Study the drawing (mm; zero at the part's minimum x, y, z) and answer. Round coordinates to 2 decimals unless told otherwise and drop trailing zeros. Write each loop counter-clockwise with the first axis right and the second up, starting at its lowest first coordinate (ties: lowest second). Pieces come first, ordered by that corner, then holes. Notation, with made-up numbers: (-2.75, -4.5) - (4.25, -4.5) arc R15 ccw to (4.25, 8.5) - close; hole circle Ø3 at (73.25, -4). An arc over 180 degrees is marked (long way). Return JSON: item names as keys, results as strings. Group by question number.
(1) Find the intervals of material crossed by line 1 along Z through (x, y) = (49.4, 3.05); line 2 along Z through (x, y) = (49.4, 1.95); line 3 along X through (y, z) = (1.95, 51), in increasing order. Write a range as [from, to].
(2) Section A-A, the plane x = 4 is taken. Write down the section's boundary in (y, z).
(3) Section D-D, the plane x = 16.5 is taken. Write down the section's boundary in (y, z), then the cut area to 3 significant figures.
(4) Section C-C, the plane x = 49.4 is taken. Write down the section's boundary in (y, z), then the cut area to 3 significant figures.
(5) Each of these flat-tipped pins is pushed along its axis until it touches: pin 1 (3.5 mm diameter, centred on x = 49.4, z = 55.8, fed in from +Y); pin 2 (8 mm diameter, centred on x = 47, z = 43.5, fed in from -Y); pin 3 (0.6 mm diameter, centred on x = 2, y = 3, fed in from +Z); pin 4 (0.8 mm diameter, centred on y = 2.5, z = 55, fed in from -X). Where does it stop, or does it pass through?
(6) Section B-B, the plane z = 27.5 is taken. Write down the section's boundary in (x, y), then the cut area to 3 significant figures.
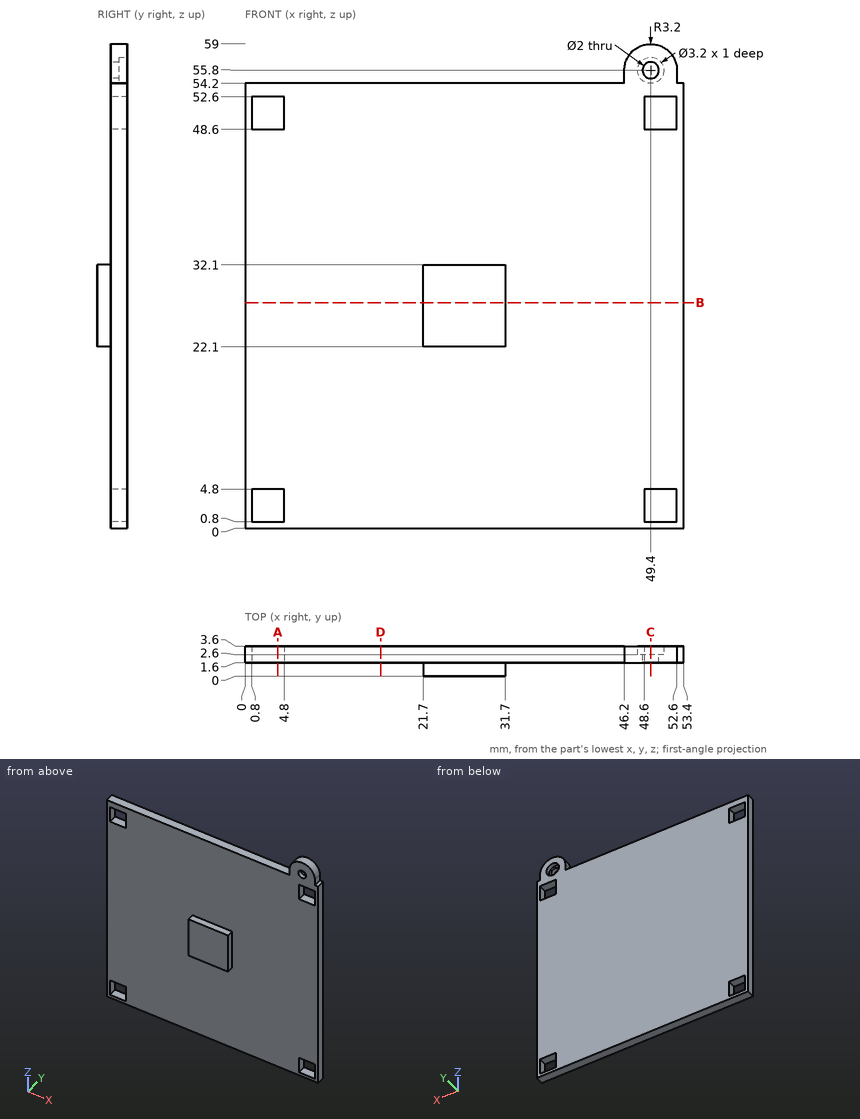
Working result:
{
 "1": {"line 1": "z = [0, 0.8], [4.8, 48.6], [52.6, 54.2], [57.4, 59]", "line 2": "z = [0, 0.8], [4.8, 48.6], [52.6, 54.8], [56.8, 59]", "line 3": "x = [0, 0.8], [4.8, 48.6], [52.6, 53.4]"},
 "2": {"outline": "(1.6, 0) - (3.6, 0) - (3.6, 0.8) - (1.6, 0.8) - close; (1.6, 4.8) - (3.6, 4.8) - (3.6, 48.6) - (1.6, 48.6) - close; (1.6, 52.6) - (3.6, 52.6) - (3.6, 54.2) - (1.6, 54.2) - close"},
 "3": {"outline": "(1.6, 0) - (3.6, 0) - (3.6, 54.2) - (1.6, 54.2) - close", "area": "108 mm^2"},
 "4": {"outline": "(1.6, 0) - (3.6, 0) - (3.6, 0.8) - (1.6, 0.8) - close; (1.6, 4.8) - (3.6, 4.8) - (3.6, 48.6) - (1.6, 48.6) - close; (1.6, 52.6) - (3.6, 52.6) - (3.6, 54.2) - (2.6, 54.2) - (2.6, 54.8) - (1.6, 54.8) - close; (1.6, 56.8) - (2.6, 56.8) - (2.6, 57.4) - (3.6, 57.4) - (3.6, 59) - (1.6, 59) - close", "area": "96.8 mm^2"},
 "5": {"pin 1": "stops at y = 3.6", "pin 2": "stops at y = 1.6", "pin 3": "stops at z = 54.2", "pin 4": "stops at x = 46.2"},
 "6": {"outline": "(0, 1.6) - (21.7, 1.6) - (21.7, 0) - (31.7, 0) - (31.7, 1.6) - (53.4, 1.6) - (53.4, 3.6) - (0, 3.6) - close", "area": "123 mm^2"}
}
